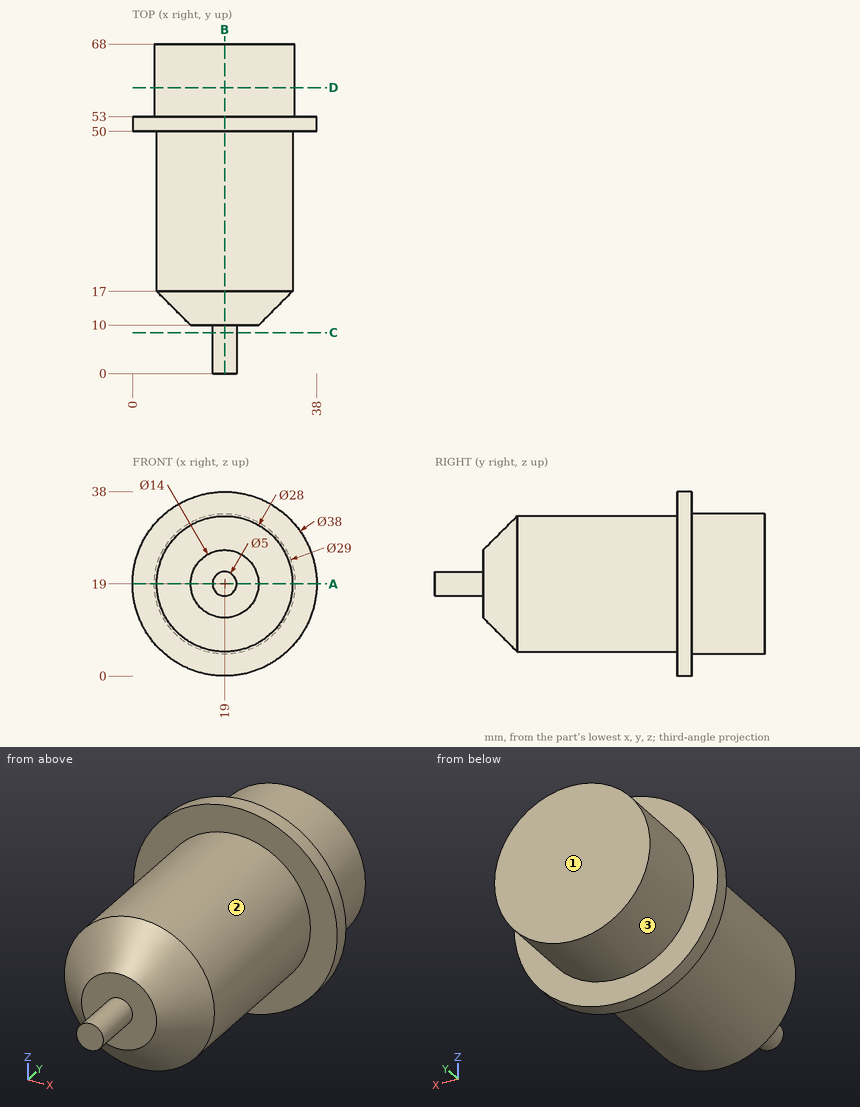
Verification items for this drawing (mm, ordinates from the low corner). A direction names the side the tool comes from. Give positions to 0.01 mm unless a question says otherwise; leave off trailing zeros. Loops run counter-clockwise (first coordinate to the right, second up) from the corner with the lowest first, then second, coordinate; pieces in that order, holes last. Notation, with made-up numbers: M 36.25,3 L 75.25,3 A24 cw 75.25,26 Z; hole C 81,17 d5. An arc over 180 degrees is marked long. Answer as a JSON object with one key per item and string values. Group by question number.
Q1. Cross-section at D-D on y = 59. Record the cut outline in (x, z), then the cut area to 3 significant figures.
Q2. Material ranges on line 1 along Z through (x, y) = (19, 33); line 2 along X through (y, z) = (31, 18.5); line 3 along Y through (x, z) = (12, 10.5), recorded low to high. Write a range as [from, to].
Q3. Access from +Z, -Z, +X, -X, +Y, -Y to the whole of each face (thin tool, end or side, straight path). Record for the marked faces 1, 2 and 3.
Q4. Cross-section at C-C on y = 8.5. Record the cut outline in (x, z).
Q5. Cross-section at B-B on x = 19. Record the cut outline in (y, z).
Q6. Go/stop test with flat-tipped pins: P1, Ø1.5, axis at y = 22, z = 30, coming from the +X side; P2, Ø1, axis at x = 28.5, z = 13.5, coming from the -Y side; P3, Ø3, axis at x = 29.5, y = 60.5, coming from the -Z side. Record where each tip stops, or that it passes through.
Q7. Cross-section at A-A on z = 19. Record the cut outline in (x, y), then the cut area to 3 significant figures.
Evaluation:
{
 "1": {"outline": "C 19,19 d29", "area": "661 mm2"},
 "2": {"line 1": "z = [5, 33]", "line 2": "x = [5.01, 32.99]", "line 3": "y = [14.01, 68]"},
 "3": {"face 1": "+Z, -Z, +X, -X, +Y", "face 2": "-Y", "face 3": "+Y"},
 "4": {"outline": "C 19,19 d5"},
 "5": {"outline": "M 0,16.5 L 10,16.5 L 10,12 L 17,5 L 50,5 L 50,0 L 53,0 L 53,4.5 L 68,4.5 L 68,33.5 L 53,33.5 L 53,38 L 50,38 L 50,33 L 17,33 L 10,26 L 10,21.5 L 0,21.5 Z"},
 "6": {"P1": "stops at x = 28.54", "P2": "stops at y = 13.48", "P3": "stops at z = 7.63"},
 "7": {"outline": "M 0,50 L 5,50 L 5,17 L 12,10 L 16.5,10 L 16.5,0 L 21.5,0 L 21.5,10 L 26,10 L 33,17 L 33,50 L 38,50 L 38,53 L 33.5,53 L 33.5,68 L 4.5,68 L 4.5,53 L 0,53 Z", "area": "1,670 mm2"}
}
